```python
from build123d import *

# Parameters (mm, degrees)
BOSS_EXTRUDE1_DEPTH      = 75
BOSS_EXTRUDE1_DEPTH_BACK = 75
CUT_EXTRUDE1_REACH       = 78.609
SKETCH2_R                = 2.5
SKETCH2_R_2              = 2.75
CHAMFER1_SIZE            = 3.5
SKETCH3_W                = 6.2
SKETCH3_H                = 4
CUT_EXTRUDE2_DEPTH       = 35
CHAMFER3_SIZE            = 0.5
FILLET1_R                = 1
CHAMFER2_SIZE            = 0.5


with BuildPart() as part:
    # Sketch1 → Boss-Extrude1 (new, two sides: drawn at the far end of the back side and taken through both)
    with BuildSketch(Plane.XY.offset(-BOSS_EXTRUDE1_DEPTH_BACK)):
        Polygon((0, 0), (7.6, 0), (7.6, -5), (10, -5), (10, 7), (-10, 7), (-10, -5), (-7.6, -5), (-7.6, 0), align=None)
    extrude(amount=BOSS_EXTRUDE1_DEPTH + BOSS_EXTRUDE1_DEPTH_BACK)

    # Sketch2 → Cut-Extrude1 (cut, up to next)
    with BuildSketch(Plane(origin=(0, 7, 0), x_dir=(1, 0, 0), z_dir=(0, 1, 0)), mode=Mode.PRIVATE) as cut_extrude1_sk1:
        with Locations(Location((0, -51.5, 0), (0, 0, 180))):
            Circle(SKETCH2_R)
    cut_extrude1_tool1 = extrude(cut_extrude1_sk1.sketch, amount=-CUT_EXTRUDE1_REACH, mode=Mode.PRIVATE) & part.part
    # Sketch2 → Cut-Extrude1 (cut, up to next)
    with BuildSketch(Plane(origin=(0, 7, 0), x_dir=(1, 0, 0), z_dir=(0, 1, 0)), mode=Mode.PRIVATE) as cut_extrude1_sk2:
        with Locations(Location((0, 12.7, 0), (0, 0, 180))):
            Circle(SKETCH2_R_2)
    cut_extrude1_tool2 = extrude(cut_extrude1_sk2.sketch, amount=-CUT_EXTRUDE1_REACH, mode=Mode.PRIVATE) & part.part
    # Sketch2 → Cut-Extrude1 (cut, up to next)
    with BuildSketch(Plane(origin=(0, 7, 0), x_dir=(1, 0, 0), z_dir=(0, 1, 0)), mode=Mode.PRIVATE) as cut_extrude1_sk3:
        with Locations(Location((0, -12.7, 0), (0, 0, 180))):
            Circle(SKETCH2_R_2)
    cut_extrude1_tool3 = extrude(cut_extrude1_sk3.sketch, amount=-CUT_EXTRUDE1_REACH, mode=Mode.PRIVATE) & part.part
    # Sketch2 → Cut-Extrude1 (cut, up to next)
    with BuildSketch(Plane(origin=(0, 7, 0), x_dir=(1, 0, 0), z_dir=(0, 1, 0)), mode=Mode.PRIVATE) as cut_extrude1_sk4:
        with Locations(Location((0, 51.5, 0), (0, 0, 180))):
            Circle(SKETCH2_R)
    cut_extrude1_tool4 = extrude(cut_extrude1_sk4.sketch, amount=-CUT_EXTRUDE1_REACH, mode=Mode.PRIVATE) & part.part
    add(cut_extrude1_tool1.solids().sort_by_distance((0, 7, 51.5))[0], mode=Mode.SUBTRACT)
    add(cut_extrude1_tool2.solids().sort_by_distance((0, 7, -12.7))[0], mode=Mode.SUBTRACT)
    add(cut_extrude1_tool3.solids().sort_by_distance((0, 7, 12.7))[0], mode=Mode.SUBTRACT)
    add(cut_extrude1_tool4.solids().sort_by_distance((0, 7, -51.5))[0], mode=Mode.SUBTRACT)

    # Chamfer1
    chamfer1_edges = [part.edges().sort_by_distance(p)[0] for p in [
        (2.5, 7, 51.5),
        (2.5, 7, -51.5),
    ]]
    chamfer(chamfer1_edges, length=CHAMFER1_SIZE)

    # Sketch3 → Cut-Extrude2 (cut)
    with BuildSketch(Plane.XY.offset(75)):
        with Locations((0, 2)):
            Rectangle(SKETCH3_W, SKETCH3_H)
    cut_extrude2 = extrude(amount=-CUT_EXTRUDE2_DEPTH, mode=Mode.SUBTRACT)

    # Mirror2: Cut-Extrude2 across plane
    add(cut_extrude2.mirror(Plane.XY), mode=Mode.SUBTRACT)

    # Chamfer3
    chamfer3_edges = [part.edges().sort_by_distance(p)[0] for p in [
        (2.75, 0, 12.7),
        (2.75, 7, 12.7),
        (2.75, 0, -12.7),
        (2.75, 7, -12.7),
    ]]
    chamfer(chamfer3_edges, length=CHAMFER3_SIZE)

    # Fillet1
    fillet1_edges = [part.edges().sort_by_distance(p)[0] for p in [
        (-3.1, 2, 40),
        (3.1, 2, 40),
        (-3.1, 2, -40),
        (3.1, 2, -40),
    ]]
    fillet(fillet1_edges, radius=FILLET1_R)

    # Chamfer2
    chamfer2_edges = [part.edges().sort_by_distance(p)[0] for p in [
        (-3.1, 0, -58),
        (0, 0, -40),
        (3.1, 0, -58),
        (0, 0, 40),
        (-3.1, 0, 58),
        (3.1, 0, 58),
        (-2.807106781, 0, -40.292893219),
        (2.807106781, 0, -40.292893219),
        (-2.807106781, 0, 40.292893219),
        (2.807106781, 0, 40.292893219),
    ]]
    chamfer(chamfer2_edges, length=CHAMFER2_SIZE)


solid = part.part
```
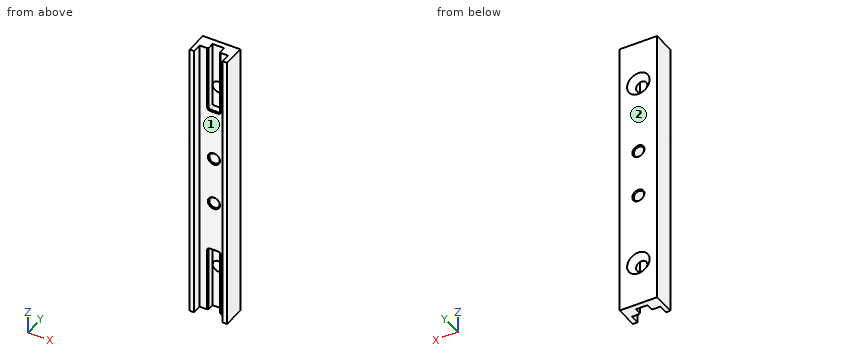
Input: part model. Units: mm. Frame: model coordinates. Face numbers are marked on the shaded views. A direction names the side the tool comes from. Coordinates: 2 decimals unless noted, no trailing zeros. Order: outer loops, then holes, each group sorted by start corner. A loop starts at its lowest first (then second) coordinate and runs counter-clockwise, first axis right, second up. Notation, with made-up numbers: (-36, 57.5) - (-9, 57.5) arc R24 ccw to (-9, 84.5) - close; hole circle Ø11 at (44.25, 29). An arc over 180 degrees is marked (long way). Return JSON: item names as keys, results as strings.
Q1. Cut plane D-D (z = 12.7). Return loops of the section in (x, y), then the cut area to 3 significant figures.
The answers:
{"outline": "(-10, -5) - (-7.6, -5) - (-7.6, 0) - (-3.25, 0) - (-2.75, 0.5) - (-2.75, 6.5) - (-3.25, 7) - (-10, 7) - close; (2.75, 0.5) - (3.25, 0) - (7.6, 0) - (7.6, -5) - (10, -5) - (10, 7) - (3.25, 7) - (2.75, 6.5) - close", "area": "125 mm2"}
Q2. First-contact query: pin 1 (3 mm diameter, centred on x = 5, z = -57.5, fed in from -Y); pin 2 (7 mm diameter, centred on x = 0, z = -51.5, fed in from -Y); pin 3 (1 mm diameter, centred on x = 0, y = 2.5, fed in from -Z); pin 4 (12 mm diameter, centred on x = -3.5, z = 14, fed in from -Y). Flat tips, straight axial feed; report the tip coordinate or a pass-through.
The answers:
{"pin 1": "stops at y = 0", "pin 2": "stops at y = 0.1", "pin 3": "stops at z = -40", "pin 4": "stops at y = -5"}
Q3. Ray query, probe 1 along Z at (x, y) = (0, 3.45); probe 2 along X at (y, z) = (3.25, 42.5); probe 3 along X at (y, z) = (-1.75, 49). Return the intervals inside material, ascending.
The answers:
{"probe 1": "z = -40 to -15.45, -9.95 to 9.95, 15.45 to 40", "probe 2": "x = -10 to -3.1, 3.1 to 10", "probe 3": "x = -10 to -7.6, 7.6 to 10"}
Q4. Cut plane C-C (z = -36). Return loops of the section in (x, y).
The answers:
{"outline": "(-10, -5) - (-7.6, -5) - (-7.6, 0) - (7.6, 0) - (7.6, -5) - (10, -5) - (10, 7) - (-10, 7) - close"}
Q5. Cut plane B-B (z = -51.5). Return loops of the section in (x, y), then the cut area to 3 significant figures.
The answers:
{"outline": "(-10, -5) - (-7.6, -5) - (-7.6, 0) - (-3.6, 0) - (-3.1, 0.5) - (-3.1, 4) - (-3, 4) - (-6, 7) - (-10, 7) - close; (3, 4) - (3.1, 4) - (3.1, 0.5) - (3.6, 0) - (7.6, 0) - (7.6, -5) - (10, -5) - (10, 7) - (6, 7) - close", "area": "112 mm2"}
Q6. Access query for the marked faces 1 and 2. Directions: +Z, -Z, +X, -X, +Y, -Y. A direction counts if a zero-diameter tool reaches every point of the face in a straight line with its end or side. Return the directions, or none.
The answers:
{"face 1": "+Z, -Z, -Y", "face 2": "+Z, -Z, +X, -X, +Y"}
Q7. Cut plane A-A (x = 0). State how many separate pieces and enclosed holes the cut face has, then the cut area to 3 significant figures.
The answers:
{"separate pieces": "5", "enclosed holes": "0", "area": "638 mm2"}
